Input: part model. Units: mm. Frame: model coordinates. A direction names the side the tool comes from. Round coordinates to 2 decimals unless told otherwise and drop trailing zeros. Loops run counter-clockwise (first coordinate to the right, second up) from the corner with the lowest first, then second, coordinate; pieces in that order, holes last. Notation, with made-up numbers: (42, -5) - (47, -5) arc R5 ccw to (47, 4) - close; hole circle Ø11 at (22, 17.5). An arc over 180 degrees is marked (long way). One line per question, with ' | ' between items. Start each with the question number.
Autodesk Inventor part; units mm, degrees
ref_plane "YZ Plane" through (0, 0, 0) normal (1, 0, 0) x (0, 1, 0)
ref_plane "XZ Plane" through (0, 0, 0) normal (0, 1, 0) x (-1, 0, 0)
ref_plane "XY Plane" through (0, 0, 0) normal (0, 0, 1) x (1, 0, 0)
sketch "Эскиз1" plane through (0, 0, 0) normal (0, 0, 1) x (1, 0, 0)
  circle A0 centre (0, 0) radius 10
  dimension "d0" = 20
extrude "Выдавливание1" add sketch "Эскиз1" along normal blind 2
sketch "Эскиз2" plane through (0, 0, 0) normal (0, 0, -1) x (-1, 0, 0)
  circle A0 centre (0, 0) radius 3 construction
  line L0 (1.7321, 3) -> (3.4641, 0)
  line L1 (3.4641, 0) -> (1.7321, -3)
  line L2 (1.7321, -3) -> (-1.7321, -3)
  line L3 (-1.7321, -3) -> (-3.4641, 0)
  line L4 (-3.4641, 0) -> (-1.7321, 3)
  line L5 (-1.7321, 3) -> (1.7321, 3)
  point P0 (0, 3)
  dimension "d3" = 6
extrude "Выдавливание2" cut sketch "Эскиз2" against normal blind 1.5
sketch "Эскиз3" plane through (0, 0, 1.5) normal (0, 0, -1) x (-1, 0, 0)
  circle A0 centre (0, 0) radius 1.75
  dimension "d6" = 3.5
extrude "Выдавливание3" cut sketch "Эскиз3" against normal blind 10
properties part number "hand2"
(1) Pin query (flat end, axial travel): P1, Ø2, axis at x = 0, y = 0, coming from the -Z side. Return the tip coordinate at first contact, or that it passes through.
(2) Pull-direction query (X, two-part tool) for faces 1 (the face through (-2.17, 9.76, 0.99)), 2 (the face through (-2.4, 2.4, 0)), 3 (the face through (0, 3, 1)); classes: released by +X, released by -X, zero draft, split by the parting line, or undercut.
(3) Line query: line 1 along Y through (x, z) = (0, 1.8); line 2 along Y through (x, z) = (-0.75, 0.9); line 3 along Z through (x, y) = (1.5, 2.75). Output: solid intervals per line, ascending. Write a range as from..to.
(4) Section A-A, the plane z = 0.65. Output: boundary loops of the cut face in (x, y), plus the area to 3 significant figures.
(5) Section D-D, the plane x = 4.5. Output: boundary loops of the cut face in (y, z).
(6) Section B-B, the plane x = 0. Output: boundary loops of the cut face in (y, z), plus the area to 4 significant figures.
(7) Reachability of faces 4 (the face through (-1.5, 1.4, 1.5)), 5 (the face through (-1.617, -0.67, 1.746)) from +Z, -Z, +X, -X, +Y, -Y: full face, straight path, thin tool, end or side. Return the list, or none.
(8) Section C-C, the plane y = -6. Output: boundary loops of the cut face in (x, z), plus the area to 3 significant figures.
Derived:
1) P1: passes through
2) face 1: split by the parting line | face 2: zero draft | face 3: undercut
3) line 1: y = -10..-1.75, 1.75..10 | line 2: y = -9.97..-3, 3..9.97 | line 3: z = 1.5..2
4) outline: circle Ø20 at (0, 0); hole (-3.46, 0) - (-1.73, -3) - (1.73, -3) - (3.46, 0) - (1.73, 3) - (-1.73, 3) - close | area: 283 mm²
5) outline: (-8.93, 0) - (8.93, 0) - (8.93, 2) - (-8.93, 2) - close
6) outline: (-10, 0) - (-3, 0) - (-3, 1.5) - (-1.75, 1.5) - (-1.75, 2) - (-10, 2) - close; (1.75, 1.5) - (3, 1.5) - (3, 0) - (10, 0) - (10, 2) - (1.75, 2) - close | area: 29.25 mm²
7) face 4: -Z | face 5: +Z, -Z
8) outline: (-8, 0) - (8, 0) - (8, 2) - (-8, 2) - close | area: 32.0 mm²
